CAD build for the part. Positions are in the model's coordinates, mm. A direction names the side the tool comes from. Give positions to 0.01 mm unless a question says otherwise; leave off trailing zeros. Write each loop counter-clockwise with the first axis right and the second up, starting at its lowest first coordinate (ties: lowest second). Pieces come first, ordered by that corner, then holes. Notation, with made-up numbers: (26.5, 18) - (34.5, 18) arc R9 ccw to (34.5, 34) - close; hole circle Ø10 at (32, -16.75). An arc over 180 degrees is marked (long way). Write item = value, one per line. Start each with the question number.
```python
from build123d import *

# Parameters (mm, degrees)
SKETCH1_W           = 79.375
SKETCH1_H           = 21.209
SKETCH1_W_2         = 61.595
SKETCH1_H_2         = 3.429
BOSS_EXTRUDE1_DEPTH = 0.8
FILLET1_R           = 1.27
FILLET2_R           = 7.62
BOSS_EXTRUDE2_START = 13.97
BOSS_EXTRUDE2_DEPTH = 13.97
BOSS_EXTRUDE3_START = 0.8
BOSS_EXTRUDE3_DEPTH = 0.8


with BuildPart() as part:
    # Sketch1 → Boss-Extrude1 (new body)
    with BuildSketch(Plane(origin=(0, 0, 0), x_dir=(1, 0, 0), z_dir=(0, 1, 0))):
        Rectangle(SKETCH1_W, SKETCH1_H)
        Rectangle(SKETCH1_W_2, SKETCH1_H_2, mode=Mode.SUBTRACT)
    extrude(amount=BOSS_EXTRUDE1_DEPTH)

    # Fillet1
    fillet1_edges = [part.edges().sort_by_distance(p)[0] for p in [
        (30.7975, 0.4, 1.7145),
        (30.7975, 0.4, -1.7145),
        (-30.7975, 0.4, -1.7145),
        (-30.7975, 0.4, 1.7145),
    ]]
    fillet(fillet1_edges, radius=FILLET1_R)

    # Fillet2
    fillet2_edges = [part.edges().sort_by_distance(p)[0] for p in [
        (39.6875, 0.4, 10.6045),
        (-39.6875, 0.4, 10.6045),
        (-39.6875, 0.4, -10.6045),
        (39.6875, 0.4, -10.6045),
    ]]
    fillet(fillet2_edges, radius=FILLET2_R)

    # Sketch2 → Boss-Extrude2 (add)
    with BuildSketch(Plane(origin=(0, 0.8, 0), x_dir=(1, 0, 0), z_dir=(0, 1, 0)).offset(BOSS_EXTRUDE2_START)):
        with BuildLine():
            Line((29.5275, 2.5145), (-29.5275, 2.5145))
            ThreePointArc((-29.5275, 2.5145), (-30.991211037, 1.908211037), (-31.5975, 0.4445))
            Line((-31.5975, 0.4445), (-31.5975, -0.4445))
            ThreePointArc((-31.5975, -0.4445), (-30.991211037, -1.908211037), (-29.5275, -2.5145))
            Line((-29.5275, -2.5145), (29.5275, -2.5145))
            ThreePointArc((29.5275, -2.5145), (30.991211037, -1.908211037), (31.5975, -0.4445))
            Line((31.5975, -0.4445), (31.5975, 0.4445))
            ThreePointArc((31.5975, 0.4445), (30.991211037, 1.908211037), (29.5275, 2.5145))
        make_face()
        with BuildLine():
            Line((30.7975, -0.4445), (30.7975, 0.4445))
            ThreePointArc((30.7975, 0.4445), (30.425525612, 1.342525612), (29.5275, 1.7145))
            Line((29.5275, 1.7145), (-29.5275, 1.7145))
            ThreePointArc((-29.5275, 1.7145), (-30.425525612, 1.342525612), (-30.7975, 0.4445))
            Line((-30.7975, 0.4445), (-30.7975, -0.4445))
            ThreePointArc((-30.7975, -0.4445), (-30.425525612, -1.342525612), (-29.5275, -1.7145))
            Line((-29.5275, -1.7145), (29.5275, -1.7145))
            ThreePointArc((29.5275, -1.7145), (30.425525612, -1.342525612), (30.7975, -0.4445))
        make_face(mode=Mode.SUBTRACT)
    extrude(amount=-BOSS_EXTRUDE2_DEPTH)

    # Sketch3 → Boss-Extrude3 (add)
    with BuildSketch(Plane(origin=(0, 14.77, 0), x_dir=(1, 0, 0), z_dir=(0, 1, 0)).offset(BOSS_EXTRUDE3_START)):
        with BuildLine():
            Line((-32.0675, -10.6045), (32.0675, -10.6045))
            ThreePointArc((32.0675, -10.6045), (37.455653673, -8.372653673), (39.6875, -2.9845))
            Line((39.6875, -2.9845), (39.6875, 2.9845))
            ThreePointArc((39.6875, 2.9845), (37.455653673, 8.372653673), (32.0675, 10.6045))
            Line((32.0675, 10.6045), (-32.0675, 10.6045))
            ThreePointArc((-32.0675, 10.6045), (-37.455653673, 8.372653673), (-39.6875, 2.9845))
            Line((-39.6875, 2.9845), (-39.6875, -2.9845))
            ThreePointArc((-39.6875, -2.9845), (-37.455653673, -8.372653673), (-32.0675, -10.6045))
        make_face()
        with BuildLine():
            Line((29.5275, 1.7145), (-29.5275, 1.7145))
            ThreePointArc((-29.5275, 1.7145), (-30.425525612, 1.342525612), (-30.7975, 0.4445))
            Line((-30.7975, 0.4445), (-30.7975, -0.4445))
            ThreePointArc((-30.7975, -0.4445), (-30.425525612, -1.342525612), (-29.5275, -1.7145))
            Line((-29.5275, -1.7145), (29.5275, -1.7145))
            ThreePointArc((29.5275, -1.7145), (30.425525612, -1.342525612), (30.7975, -0.4445))
            Line((30.7975, -0.4445), (30.7975, 0.4445))
            ThreePointArc((30.7975, 0.4445), (30.425525612, 1.342525612), (29.5275, 1.7145))
        make_face(mode=Mode.SUBTRACT)
    extrude(amount=-BOSS_EXTRUDE3_DEPTH)


solid = part.part
```
1. Tool access for faces 1 (the cylindrical face through (31, 7.9, 1.9)), 2 (the flat face through (0, 8, 2.514)), 3 (the cylindrical face through (31, 7.9, -1.9)), 4 (the cylindrical face through (-30.42, 7.89, -1.35)): list every direction of +Z, -Z, +X, -X, +Y, -Y with a clear straight run to the whole face (end or side of a thin tool).
2. Cut at A-A (x = 27). Give the cut face in (y, z).
3. Cut at B-B (y = 13). Give the cut face in (x, z), then the cut area to 3 significant figures.
4. Wall check: line 1 along Z through (x, y) = (-13.5, 5); line 2 along Y through (x, z) = (-10.5, 4); line 3 along X through (y, z) = (11.25, 1.5). Give the ranges that are in metal, low to high.
5. Cut at C-C (z = 6.5). Give the cut face in (x, y).
6. Pin check, flat tips, straight feed: pin 1 Ø1 at (y, z) = (11.5, 0) entering from +X; pin 2 Ø3 at (x, y) = (-21.5, 13) entering from -Z; pin 3 Ø2 at (y, z) = (5, 2) entering from +X. Stop position of each tip, or through.
7. Mould opens along Y. For faces 5 (the cylindrical face through (-31, 7.9, 1.9)), 6 (the flat face through (0, 8, 1.714)), 7 (the flat face through (-1, 15.57, -3)) say: +Y half, -Y half, draft (parallel to the pull), parting line (faces both ways), or undercut.
8. Cut at D-D (z = -5.5). Give the cut face in (x, y).
Output:
q1.face_1 = +Z, +X
q1.face_2 = +Z, +X, -X
q1.face_3 = -Z, +X
q1.face_4 = +Y, -Y
q2.outline = (0, -10.6) - (0.8, -10.6) - (0.8, -2.51) - (14.77, -2.51) - (14.77, -10.6) - (15.57, -10.6) - (15.57, -1.71) - (0, -1.71) - close; (0, 1.71) - (15.57, 1.71) - (15.57, 10.6) - (14.77, 10.6) - (14.77, 2.51) - (0.8, 2.51) - (0.8, 10.6) - (0, 10.6) - close
q3.outline = (-31.6, -0.44) arc R2.07 ccw to (-29.53, -2.51) - (29.53, -2.51) arc R2.07 ccw to (31.6, -0.44) - (31.6, 0.44) arc R2.07 ccw to (29.53, 2.51) - (-29.53, 2.51) arc R2.07 ccw to (-31.6, 0.44) - close; hole (-30.8, -0.44) arc R1.27 ccw to (-29.53, -1.71) - (29.53, -1.71) arc R1.27 ccw to (30.8, -0.44) - (30.8, 0.44) arc R1.27 ccw to (29.53, 1.71) - (-29.53, 1.71) arc R1.27 ccw to (-30.8, 0.44) - close
q3.area = 104 mm2
q4.line_1 = -2.51 to -1.71, 1.71 to 2.51
q4.line_2 = 0 to 0.8, 14.77 to 15.57
q4.line_3 = -31.31 to -30.23, 30.23 to 31.31
q5.outline = (-38.83, 0) - (38.83, 0) - (38.83, 0.8) - (-38.83, 0.8) - close; (-38.83, 14.77) - (38.83, 14.77) - (38.83, 15.57) - (-38.83, 15.57) - close
q6.pin_1 = 31.6
q6.pin_2 = -2.51
q6.pin_3 = 31.52
q7.face_5 = undercut
q7.face_6 = draft
q7.face_7 = +Y half
q8.outline = (-39.26, 0) - (39.26, 0) - (39.26, 0.8) - (-39.26, 0.8) - close; (-39.26, 14.77) - (39.26, 14.77) - (39.26, 15.57) - (-39.26, 15.57) - close
